Here's how the part is built. I have some questions about the finished solid (model axes, mm). Face numbers are marked on the shaded views. A direction names the side the tool comes from. Coordinates: 2 decimals unless noted, no trailing zeros. Write each loop counter-clockwise with the first axis right and the second up, starting at its lowest first coordinate (ties: lowest second). Pieces come first, ordered by that corner, then holes.
```python
from build123d import *

# Parameters (mm, degrees)
SKETCH1_R           = 1.625
BOSS_EXTRUDE1_DEPTH = 2
SKETCH1_3_R         = 3.9
BOSS_EXTRUDE2_DEPTH = 2
FILLET1_R           = 1


with BuildPart() as part:
    # Sketch1 → Boss-Extrude1 (new body)
    with BuildSketch(Plane(origin=(0, 0, 0), x_dir=(1, 0, 0), z_dir=(0, 1, 0))):
        with BuildLine():
            ThreePointArc((-3.619822402, -7.693676988), (0, -11.125), (3.619822402, -7.693676988))
            ThreePointArc((3.619822402, -7.693676988), (4.048280274, -5.285374691), (5.048596372, -3.053141771))
            ThreePointArc((5.048596372, -3.053141771), (0, 5.9), (-5.048596372, -3.053141771))
            ThreePointArc((-5.048596372, -3.053141771), (-4.048280274, -5.285374691), (-3.619822402, -7.693676988))
        make_face()
        with Locations(Location((0, -7.5, 0), (0, 0, 270))):
            Circle(SKETCH1_R, mode=Mode.SUBTRACT)
    extrude(amount=BOSS_EXTRUDE1_DEPTH)

    # Sketch1_3 → Boss-Extrude2 (add)
    with BuildSketch(Plane(origin=(0, 0, 0), x_dir=(1, 0, 0), z_dir=(0, 1, 0))):
        with Locations(Location((0, 0, 0), (0, 0, 270))):
            Circle(SKETCH1_3_R)
    extrude(amount=-BOSS_EXTRUDE2_DEPTH)

    # Fillet1
    fillet1_edges = [part.edges().sort_by_distance(p)[0] for p in [
        (0, -2, -3.9),
    ]]
    fillet(fillet1_edges, radius=FILLET1_R)


solid = part.part
```
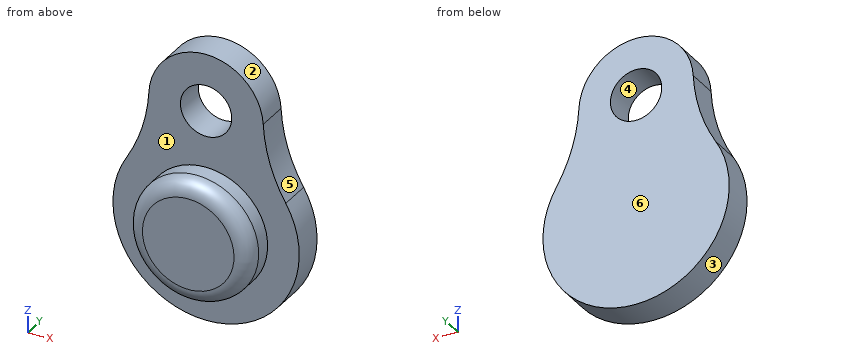
1) Imagine slicing it at C-C on z = 0. Please give me the cut outline in (x, y), then the cut area to 3 significant figures.
Values follow:
outline: (-5.9, 0) - (-3.9, 0) - (-3.9, -1) arc R1 ccw to (-2.9, -2) - (2.9, -2) arc R1 ccw to (3.9, -1) - (3.9, 0) - (5.9, 0) - (5.9, 2) - (-5.9, 2) - close
area: 38.8 mm2
2) Imagine slicing it at B-B on y = 1.2. Please give me the cut outline in (x, z) (3 decimals), then the cut area to 3 significant figures.
Values follow:
outline: (-5.049, 3.053) arc R5.9 ccw (long way) to (5.049, 3.053) arc R10 cw to (3.62, 7.694) arc R3.625 ccw to (-3.62, 7.694) arc R10 cw to start; hole circle Ø3.25 at (0, 7.5)
area: 138 mm2
3) Imagine slicing it at D-D on z = 7. Please give me the cut outline in (x, y), then the cut area to 3 significant figures.
Values follow:
outline: (-3.68, 0) - (-1.55, 0) - (-1.55, 2) - (-3.68, 2) - close; (1.55, 0) - (3.68, 0) - (3.68, 2) - (1.55, 2) - close
area: 8.54 mm2
4) On a 3-axis mill with a long thin cutter (end or side, diameter ignored), from which of +Z, -Z, +X, -X, +Y, -Y can I reach the whole of each face in a straight line? I mean the marked faces 1 and 2. Say none if no direction works.
Values follow:
face 1: -Y
face 2: +Z, +Y, -Y
5) Will this pin go through, and if not, where does the flat tip stop? pin 1 (1 mm diameter, centred on x = 1.5, y = 0, fed in from -Z).
Values follow:
pin 1: stops at z = -5.81
6) Imagine slicing it at A-A on x = 0. Please give me the cut outline in (y, z) (3 decimals), then the cut area to 3 significant figures.
Values follow:
outline: (-2, -2.9) arc R1 ccw to (-1, -3.9) - (0, -3.9) - (0, -5.9) - (2, -5.9) - (2, 5.875) - (0, 5.875) - (0, 3.9) - (-1, 3.9) arc R1 ccw to (-2, 2.9) - close; (0, 9.125) - (2, 9.125) - (2, 11.125) - (0, 11.125) - close
area: 42.7 mm2
7) We'd pull the mould along Z, two halves only. Please class the marked faces 3, 4, 5 and 6: pulls with the +Z half, pulls with the -Z half, needs draft (parallel to the pull), parting line crosses it, or undercut.
Values follow:
face 3: parting line crosses it
face 4: undercut
face 5: pulls with the +Z half
face 6: needs draft
8) I need wall thicknesses on probe 1 along Y at (x, z) = (4.5, -1); probe 2 along X at (y, z) = (0.8, 7.5) (3 decimals); probe 3 along Z at (x, y) = (-1.25, 0.9). Which ranges of each line are inside material? Lowest first, please.
Values follow:
probe 1: y = 0 to 2
probe 2: x = -3.632 to -1.625, 1.625 to 3.632
probe 3: z = -5.77 to 6.46, 8.54 to 10.9
